from build123d import *

# Parameters (mm, degrees)
EXTRUDE_1_DEPTH     = 16
SKETCH_2_W          = 56.583123952
SKETCH_2_H          = 12
CUT_EXTRUDE_1_DEPTH = 60.621829584
SKETCH_3_W          = 86.583123952
SKETCH_3_H          = 16
CUT_EXTRUDE_2_DEPTH = 60.621829584
SKETCH_4_R          = 5
CUT_EXTRUDE_3_DEPTH = 63.080693963


with BuildPart() as part:
    # 草图1 → 凸台-拉伸1 (new, symmetric)
    with BuildSketch(Plane(origin=(0, 0, 0), x_dir=(1, 0, 0), z_dir=(0, 1, 0))):
        with BuildLine():
            Line((-12.5, 45), (-12.5, -45))
            ThreePointArc((-12.5, -45), (0, -51.708438024), (12.5, -45))
            Line((12.5, -45), (12.5, 45))
            ThreePointArc((12.5, 45), (0, 51.708438024), (-12.5, 45))
        make_face()
    extrude(amount=EXTRUDE_1_DEPTH, both=True)

    # 草图2 → 切除-拉伸1 (cut, through all)
    with BuildSketch(Plane(origin=(12.5, 0, 0), x_dir=(0, 0, -1), z_dir=(1, 0, 0))):
        with Locations((-45, -6)):
            Rectangle(SKETCH_2_W, SKETCH_2_H)
    extrude(amount=-CUT_EXTRUDE_1_DEPTH, mode=Mode.SUBTRACT)

    # 草图3 → 切除-拉伸2 (cut, through all)
    with BuildSketch(Plane(origin=(12.5, 0, 0), x_dir=(0, 0, -1), z_dir=(1, 0, 0))):
        with Locations((45, 0)):
            Rectangle(SKETCH_3_W, SKETCH_3_H)
    extrude(amount=-CUT_EXTRUDE_2_DEPTH, mode=Mode.SUBTRACT)

    # 草图4 → 切除-拉伸3 (cut, through all)
    with BuildSketch(Plane(origin=(0, 16, 0), x_dir=(1, 0, 0), z_dir=(0, 1, 0))):
        with Locations(Location((0, -40, 0), (0, 0, 270))):
            Circle(SKETCH_4_R)
        with Locations(Location((0, 31, 0), (0, 0, 270))):
            Circle(SKETCH_4_R)
    extrude(amount=-CUT_EXTRUDE_3_DEPTH, mode=Mode.SUBTRACT)


solid = part.part
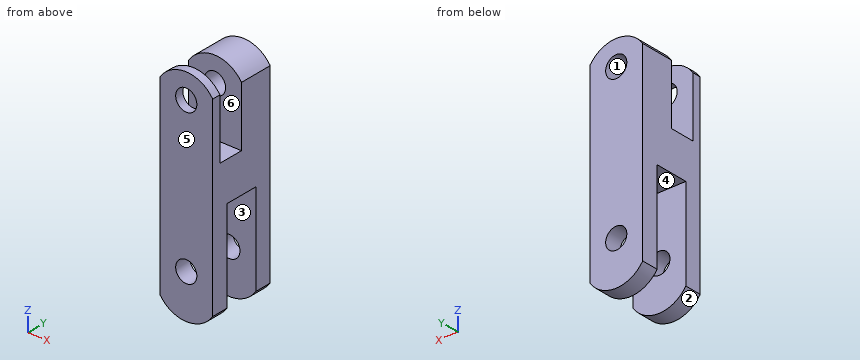
Verification items for the finished model (mm, model axes). Face numbers are marked on the shaded views. A direction names the side the tool comes from. Round coordinates to 2 decimals unless told otherwise and drop trailing zeros. Loops run counter-clockwise (first coordinate to the right, second up) from the corner with the lowest first, then second, coordinate; pieces in that order, holes last. Notation, with made-up numbers: M 13.5,30.5 L 67.5,30.5 A19 cw 67.5,53.5 Z; hole C 2.5,47.25 d6. An arc over 180 degrees is marked long. Write each question's results on one line, items separated by ' | '.
1) Section check D-D on z = -5.5. Record the boundary of the cut face in (x, y).
Checks:
outline: M -12.5,-16 L 12.5,-16 L 12.5,-8 L -12.5,-8 Z; M -12.5,8 L 12.5,8 L 12.5,16 L -12.5,16 Z
2) Section check A-A on x = 0. Record the boundary of the cut face in (y, z).
Checks:
outline: M -16,-51.71 L -8,-51.71 L -8,-36 L -16,-36 Z; M -16,-26 L -8,-26 L -8,-1.71 L 8,-1.71 L 8,-26 L 16,-26 L 16,35 L 0,35 L 0,16.71 L -12,16.71 L -12,35 L -16,35 Z; M -16,45 L -12,45 L -12,51.71 L -16,51.71 Z; M 0,45 L 16,45 L 16,51.71 L 0,51.71 Z; M 8,-51.71 L 16,-51.71 L 16,-36 L 8,-36 Z
3) Scan lines: L1, parallel to Y at x = -7.5, z = -31.5; L2, parallel to Y at x = -7, z = 46.5; L3, parallel to X at y = -13.95, z = 40. Record each from-to range of solid material in increasing order. Write a range as from..to.
Checks:
L1: y = -16..-8, 8..16 | L2: y = -16..-12, 0..16 | L3: x = -12.5..-5, 5..12.5
4) Section check C-C on y = 4. Record the boundary of the cut face in (x, z).
Checks:
outline: M -12.5,-1.71 L 12.5,-1.71 L 12.5,45 A15 ccw -12.5,45 Z; hole C 0,40 d10
5) Section check B-B on z = -31. Record the boundary of the cut face in (x, y).
Checks:
outline: M -12.5,-16 L -5,-16 L -5,-8 L -12.5,-8 Z; M -12.5,8 L -5,8 L -5,16 L -12.5,16 Z; M 5,-16 L 12.5,-16 L 12.5,-8 L 5,-8 Z; M 5,8 L 12.5,8 L 12.5,16 L 5,16 Z
6) Mould release check, pull along X, two halves, no side actions. Record for the marked faces 1, 2 and 3: released by +X, released by -X, zero draft, split by the parting line, or undercut.
Checks:
face 1: undercut | face 2: split by the parting line | face 3: zero draft
7) Access from +Z, -Z, +X, -X, +Y, -Y to the whole of each face (thin tool, end or side, straight path). Record for the marked faces 4, 5 and 6.
Checks:
face 4: -Z, +X, -X | face 5: +Z, -Z, +X, -X, -Y | face 6: +Z, +X, -X
8) Gauge pin test, flat ends, axial feed: P1, Ø4, axis at x = -2.5, y = -2.5, coming from the -Z side; P2, Ø11.5, axis at x = 0, z = -31, coming from the +Y side; P3, Ø9, axis at x = 0, z = 40, coming from the +Y side; P4, Ø3.5, axis at x = -3.5, y = -9, coming from the +Z side. Record the tip position at first contact, or that the pin passes through.
Checks:
P1: stops at z = -1.71 | P2: stops at y = 16 | P3: passes through | P4: stops at z = 16.71
